The model under review builds one solid part; all positions refer to its coordinate system, in mm. Coordinates: 2 decimals unless noted, no trailing zeros. Order: outer loops, then holes, each group sorted by start corner. A loop starts at its lowest first (then second) coordinate and runs counter-clockwise, first axis right, second up. Notation, with made-up numbers: M 17.5,27 L 29.5,27 A14 ccw 29.5,33 Z; hole C 14.5,86 d5. An arc over 180 degrees is marked long. One line per item, written item: value.
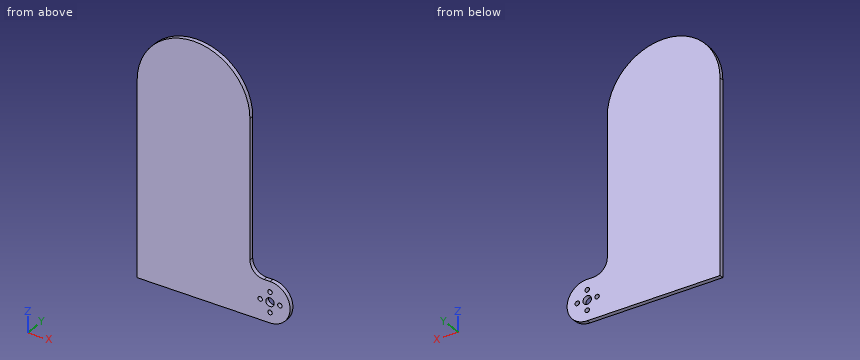
```python
from build123d import *

# Parameters (mm, degrees)
SKETCH_1_R              = 3
EXTRUDE_1_DEPTH         = 3
HOLE_WIZARD_3_2_3_2_1_D = 3.2


with BuildPart() as part:
    # 草图1 → 凸台-拉伸1 (new body)
    with BuildSketch(Plane(origin=(0, 0, 0), x_dir=(1, 0, 0), z_dir=(0, 1, 0))):
        with BuildLine():
            Line((-55.525082752, -48.428156032), (-55.525082752, 87.471843968))
            Line((-55.525082752, 87.471843968), (38.724917248, 87.471843968))
            ThreePointArc((38.724917248, 87.471843968), (52.974917248, 73.221843968), (38.724917248, 58.971843968))
            Line((38.724917248, 58.971843968), (34.474917248, 58.971843968))
            ThreePointArc((34.474917248, 58.971843968), (27.403849436, 56.04291178), (24.474917248, 48.971843968))
            Line((24.474917248, 48.971843968), (24.474917248, -48.428156032))
            ThreePointArc((24.474917248, -48.428156032), (-15.525082752, -88.428156032), (-55.525082752, -48.428156032))
        make_face()
        with Locations(Location((38.724917248, 73.221843968, 0), (0, 0, 270))):
            Circle(SKETCH_1_R, mode=Mode.SUBTRACT)
    extrude(amount=EXTRUDE_1_DEPTH)

    # Ø3.2 (3.2) 直径孔1 (through all)
    with Locations(Plane(origin=(38.724917248, 3, -80.221843968), x_dir=(0, 0, 1), z_dir=(0, 1, 0))):
        with Locations((0, 0), (7, -7), (14, 0), (7, 7)):
            Hole(HOLE_WIZARD_3_2_3_2_1_D / 2)


solid = part.part
```
(1) We need section C-C, the plane x = 1. State the section outline as (y, z) points, plus the area to 3 significant figures.
Geometry results:
outline: M 0,-87.47 L 3,-87.47 L 3,84.86 L 0,84.86 Z
area: 517 mm2
(2) We need section B-B, the plane z = -4. State the section outline as (x, y) points.
Geometry results:
outline: M -55.53,0 L 24.47,0 L 24.47,3 L -55.53,3 Z
(3) We need section A-A, the plane y = 1. State the section outline as (x, z) points.
Geometry results:
outline: M -55.53,-87.47 L 38.72,-87.47 A14.25 ccw 38.72,-58.97 L 34.47,-58.97 A10 cw 24.47,-48.97 L 24.47,48.43 A40 ccw -55.53,48.43 Z; hole C 31.72,-73.22 d3.2; hole C 38.72,-73.22 d6; hole C 38.72,-80.22 d3.2; hole C 38.72,-66.22 d3.2; hole C 45.72,-73.22 d3.2
(4) For L1, parallel to X at y = 2.8, z = 23.5; L2, parallel to X at y = 0.8, z = -75; L3, parallel to X at y = 2.05, z = -63, list the stretches that pass through material, from the lowest coordinate up.
Geometry results:
L1: x = -55.53 to 24.47
L2: x = -55.53 to 36.31, 41.14 to 52.86
L3: x = -55.53 to 48.65
(5) Insertion check: pin 1 Ø0.9 at (y, z) = (1, 14) entering from +X. The pin has a flat end and moves straight along its axis. Give the tip position at first contact, or say it passes through.
Geometry results:
pin 1: stops at x = 24.47
